```python
from build123d import *

# Parameters (mm, degrees)
SKETCH_1_W                = 180
SKETCH_1_H                = 43
EXTRUDE_335_DEPTH         = 4
SKETCH_2_R                = 5.1
SKETCH_2_R_2              = 1.6
CUT_EXTRUDE_616_DEPTH     = 5
SKETCH_10_W               = 20
SKETCH_10_H               = 43
CUT_EXTRUDE_3591_DEPTH    = 5
SKETCH_11_W               = 18
SKETCH_11_H               = 43
EXTRUDE_3904_DEPTH        = 4
SKETCH_12_W               = 40
SKETCH_12_H               = 13
CUT_EXTRUDE_3_DEPTH       = 10
SKETCH_14_R               = 1.6
CUT_EXTRUDE_4861_DEPTH    = 10
SKETCH_15_R               = 1.6
CUT_EXTRUDE_5298_DEPTH    = 5
PATTERN_LINEAR_5588_COUNT = 2
PATTERN_LINEAR_5588_PITCH = 29.8
CUT_EXTRUDE_6381_DEPTH    = 5
SKETCH_19_W               = 104
SKETCH_19_H               = 43
CUT_EXTRUDE_7034_DEPTH    = 5
FILLET_9_R                = 5
CUT_EXTRUDE_1_DEPTH       = 5
SKETCH_30_W               = 2
SKETCH_30_H               = 43
EXTRUDE_1_DEPTH           = 4
SKETCH_32_W               = 9
SKETCH_32_H               = 43
EXTRUDE_2_DEPTH           = 4
FILLET_11_R               = 5
EXTRUDE_3_DEPTH           = 4
FILLET_12_R               = 5
SKETCH_34_R               = 1.500000001
SKETCH_34_R_2             = 1.500000004
CUT_EXTRUDE_3_2_DEPTH     = 5
SKETCH_35_R               = 1.6
CUT_EXTRUDE_4_DEPTH       = 5
SKETCH_36_R               = 1.6
CUT_EXTRUDE_5_DEPTH       = 5
SKETCH_37_R               = 1.6
CUT_EXTRUDE_6_DEPTH       = 5
CUT_EXTRUDE_7_DEPTH       = 5
FILLET_15_R               = 1


with BuildPart() as part:
    # 草图1 → Extrude 335 (new body)
    with BuildSketch(Plane(origin=(0, 0, 0), x_dir=(1, 0, 0), z_dir=(0, 1, 0))):
        Rectangle(SKETCH_1_W, SKETCH_1_H)
    extrude(amount=EXTRUDE_335_DEPTH)

    # 草图2 → Cut-Extrude 616 (cut, through all)
    with BuildSketch(Plane(origin=(0, 4, 0), x_dir=(1, 0, 0), z_dir=(0, 1, 0))):
        with Locations((55, -5)):
            Circle(SKETCH_2_R)
        with Locations((63, -5)):
            Circle(SKETCH_2_R_2)
        with Locations((55, -13)):
            Circle(SKETCH_2_R_2)
        with Locations((47, -5)):
            Circle(SKETCH_2_R_2)
        with Locations((55, 3)):
            Circle(SKETCH_2_R_2)
    extrude(amount=-CUT_EXTRUDE_616_DEPTH, mode=Mode.SUBTRACT)

    # 草图10 → Cut-Extrude 3591 (cut, through all)
    with BuildSketch(Plane(origin=(0, 4, 0), x_dir=(1, 0, 0), z_dir=(0, 1, 0))):
        with Locations((80, 0)):
            Rectangle(SKETCH_10_W, SKETCH_10_H)
    extrude(amount=-CUT_EXTRUDE_3591_DEPTH, mode=Mode.SUBTRACT)

    # 草图11 → Extrude 3904 (add, through all)
    with BuildSketch(Plane(origin=(0, 4, 0), x_dir=(1, 0, 0), z_dir=(0, 1, 0))):
        with Locations((-99, 0)):
            Rectangle(SKETCH_11_W, SKETCH_11_H)
    extrude(amount=-EXTRUDE_3904_DEPTH)

    # 草图12 → Cut-Extrude 3 (cut)
    with BuildSketch(Plane(origin=(0, 4, 0), x_dir=(1, 0, 0), z_dir=(0, 1, 0))):
        with Locations((-88, -21.5)):
            Rectangle(SKETCH_12_W, SKETCH_12_H)
    extrude(amount=-CUT_EXTRUDE_3_DEPTH, mode=Mode.SUBTRACT)

    # 草图14 → Cut-Extrude 4861 (cut)
    with BuildSketch(Plane(origin=(0, 4, 0), x_dir=(1, 0, 0), z_dir=(0, 1, 0))):
        with Locations((46, -18.5)):
            Circle(SKETCH_14_R)
        with Locations((64, -18.5)):
            Circle(SKETCH_14_R)
    extrude(amount=-CUT_EXTRUDE_4861_DEPTH, mode=Mode.SUBTRACT)

    # 草图15 → Cut-Extrude 5298 (cut, through all)
    with BuildSketch(Plane(origin=(0, 4, 0), x_dir=(1, 0, 0), z_dir=(0, 1, 0))):
        with Locations((-102.9, 3.25)):
            Circle(SKETCH_15_R)
        with Locations((-73.1, 3.25)):
            Circle(SKETCH_15_R)
    extrude(amount=-CUT_EXTRUDE_5298_DEPTH, mode=Mode.SUBTRACT)

    # 草图16 → Cut-Revolve 5530 (revolve, cut)
    with BuildSketch(Plane.XY.offset(-3.25)):
        Polygon((-102.9, 0), (-99.7, 0), (-101.3, 1.6), (-102.9, 1.6), align=None)
    cut_revolve_5530 = revolve(axis=Axis((-102.9, -994.071718491, -3.25), (0, 1, 0)), mode=Mode.SUBTRACT)

    # Pattern Linear 5588: Cut-Revolve 5530 ×2
    with Locations(*[(i * PATTERN_LINEAR_5588_PITCH, 0, 0) for i in range(1, PATTERN_LINEAR_5588_COUNT)]):
        add(cut_revolve_5530, mode=Mode.SUBTRACT)

    # 草图17 → Cut-Extrude 6381 (cut, through all)
    with BuildSketch(Plane.XZ):
        with BuildLine():
            Line((-104.45, 3.75), (-101.35, 3.75))
            ThreePointArc((-101.35, 3.75), (-99.85, 5.25), (-101.35, 6.75))
            Line((-101.35, 6.75), (-101.35, 9.75))
            ThreePointArc((-101.35, 9.75), (-99.85, 11.25), (-101.35, 12.75))
            Line((-101.35, 12.75), (-104.45, 12.75))
            ThreePointArc((-104.45, 12.75), (-105.95, 11.25), (-104.45, 9.75))
            Line((-104.45, 9.75), (-104.45, 6.75))
            ThreePointArc((-104.45, 6.75), (-105.95, 5.25), (-104.45, 3.75))
        make_face()
        with BuildLine():
            Line((-104.45, -16.25), (-104.45, -13.25))
            ThreePointArc((-104.45, -13.25), (-105.95, -11.75), (-104.45, -10.25))
            Line((-104.45, -10.25), (-101.35, -10.25))
            ThreePointArc((-101.35, -10.25), (-99.85, -11.75), (-101.35, -13.25))
            Line((-101.35, -13.25), (-101.35, -16.25))
            ThreePointArc((-101.35, -16.25), (-99.85, -17.75), (-101.35, -19.25))
            Line((-101.35, -19.25), (-104.45, -19.25))
            ThreePointArc((-104.45, -19.25), (-105.95, -17.75), (-104.45, -16.25))
        make_face()
        with BuildLine():
            Line((-71.55, -16.25), (-71.55, -13.25))
            ThreePointArc((-71.55, -13.25), (-70.05, -11.75), (-71.55, -10.25))
            Line((-71.55, -10.25), (-74.65, -10.25))
            ThreePointArc((-74.65, -10.25), (-76.15, -11.75), (-74.65, -13.25))
            Line((-74.65, -13.25), (-74.65, -16.25))
            ThreePointArc((-74.65, -16.25), (-76.15, -17.75), (-74.65, -19.25))
            Line((-74.65, -19.25), (-71.55, -19.25))
            ThreePointArc((-71.55, -19.25), (-70.05, -17.75), (-71.55, -16.25))
        make_face()
        with BuildLine():
            Line((-71.55, 9.75), (-71.55, 6.75))
            ThreePointArc((-71.55, 6.75), (-70.05, 5.25), (-71.55, 3.75))
            Line((-71.55, 3.75), (-74.65, 3.75))
            ThreePointArc((-74.65, 3.75), (-76.15, 5.25), (-74.65, 6.75))
            Line((-74.65, 6.75), (-74.65, 9.75))
            ThreePointArc((-74.65, 9.75), (-76.15, 11.25), (-74.65, 12.75))
            Line((-74.65, 12.75), (-71.55, 12.75))
            ThreePointArc((-71.55, 12.75), (-70.05, 11.25), (-71.55, 9.75))
        make_face()
    extrude(amount=-CUT_EXTRUDE_6381_DEPTH, mode=Mode.SUBTRACT)

    # 草图19 → Cut-Extrude 7034 (cut, through all)
    with BuildSketch(Plane(origin=(0, 4, 0), x_dir=(1, 0, 0), z_dir=(0, 1, 0))):
        with Locations((-56, 0)):
            Rectangle(SKETCH_19_W, SKETCH_19_H)
    extrude(amount=-CUT_EXTRUDE_7034_DEPTH, mode=Mode.SUBTRACT)

    # 圆角9
    fillet_9_edges = [part.edges().sort_by_distance(p)[0] for p in [
        (-4, 2, 21.5),
        (-4, 2, -21.5),
        (70, 2, 21.5),
        (70, 2, -21.5),
    ]]
    fillet(fillet_9_edges, radius=FILLET_9_R)

    # 草图29 → Cut-Extrude 1 (cut, through all)
    with BuildSketch(Plane(origin=(0, 4, 0), x_dir=(1, 0, 0), z_dir=(0, 1, 0))):
        Polygon((1, 21.5), (10.830690118, 21.5), (10.830690118, -21.5), (1, -21.5), (-4.254253264, -21.5), (-4.254253264, 21.5), align=None)
    extrude(amount=-CUT_EXTRUDE_1_DEPTH, mode=Mode.SUBTRACT)

    # 草图30 → 凸台-拉伸1 (add)
    with BuildSketch(Plane(origin=(0, 4, 0), x_dir=(1, 0, 0), z_dir=(0, 1, 0))):
        with Locations((9.830690118, 0)):
            Rectangle(SKETCH_30_W, SKETCH_30_H)
    extrude(amount=-EXTRUDE_1_DEPTH)

    # 草图32 → Extrude 2 (add)
    with BuildSketch(Plane.XZ):
        with Locations((4.330690118, 0)):
            Rectangle(SKETCH_32_W, SKETCH_32_H)
    extrude(amount=-EXTRUDE_2_DEPTH)

    # 圆角11
    fillet_11_edges = [part.edges().sort_by_distance(p)[0] for p in [
        (-0.169309882, 2, -21.5),
        (-0.169309882, 2, 21.5),
    ]]
    fillet(fillet_11_edges, radius=FILLET_11_R)

    # 草图33 → 凸台-拉伸3 (add)
    with BuildSketch(Plane.XZ):
        Polygon((70, 16.5), (70, 25.500000005), (65, 25.500000005), (0, 25.500000005), (-0.169309882, 25.500000005), (-0.169309882, 16.5), align=None)
    extrude(amount=-EXTRUDE_3_DEPTH)

    # 圆角12
    fillet_12_edges = [part.edges().sort_by_distance(p)[0] for p in [
        (-0.169309882, 2, 25.500000005),
        (70, 2, 25.500000005),
    ]]
    fillet(fillet_12_edges, radius=FILLET_12_R)

    # 草图34 → Cut-Extrude 3 2 (cut, through all)
    with BuildSketch(Plane.XZ):
        with Locations((63.455393867, 20.5)):
            Circle(SKETCH_34_R)
        with Locations((47.301465353, 20.5)):
            Circle(SKETCH_34_R_2)
    extrude(amount=-CUT_EXTRUDE_3_2_DEPTH, mode=Mode.SUBTRACT)

    # 草图35 → 切除-拉伸4 (cut, through all)
    with BuildSketch(Plane.XZ):
        with Locations((34, 0.636740591)):
            Circle(SKETCH_35_R)
        with Locations((34, 9.1)):
            Circle(SKETCH_35_R)
    extrude(amount=-CUT_EXTRUDE_4_DEPTH, mode=Mode.SUBTRACT)

    # 草图36 → 切除-拉伸5 (cut, through all)
    with BuildSketch(Plane.XZ):
        with Locations((9.830690118, -5.9)):
            Circle(SKETCH_36_R)
        with Locations((9.830690118, 9.7)):
            Circle(SKETCH_36_R)
        with Locations((9.830690118, -16.948915218)):
            Circle(SKETCH_36_R)
        with Locations((19.830690118, -16.948915218)):
            Circle(SKETCH_36_R)
    extrude(amount=-CUT_EXTRUDE_5_DEPTH, mode=Mode.SUBTRACT)

    # 草图37 → 切除-拉伸6 (cut, through all)
    with BuildSketch(Plane(origin=(0, 4, 0), x_dir=(1, 0, 0), z_dir=(0, 1, 0))):
        with Locations((19.925091374, -9.664193429)):
            Circle(SKETCH_37_R)
    extrude(amount=-CUT_EXTRUDE_6_DEPTH, mode=Mode.SUBTRACT)

    # 草图38 → 切除-拉伸7 (cut, through all)
    with BuildSketch(Plane.XZ):
        with BuildLine():
            Line((44, 25.500000005), (44, 19.500000005))
            ThreePointArc((44, 19.500000005), (43.414213562, 18.085786442), (42, 17.500000005))
            Line((42, 17.500000005), (26, 17.500000005))
            ThreePointArc((26, 17.500000005), (24.585786438, 18.085786442), (24, 19.500000005))
            Line((24, 19.500000005), (24, 25.500000005))
            Line((24, 25.500000005), (44, 25.500000005))
        make_face()
    extrude(amount=-CUT_EXTRUDE_7_DEPTH, mode=Mode.SUBTRACT)

    # 圆角15
    fillet_15_edges = [part.edges().sort_by_distance(p)[0] for p in [
        (24, 2, 25.500000005),
        (44, 2, 25.500000005),
    ]]
    fillet(fillet_15_edges, radius=FILLET_15_R)


solid = part.part
```
Design review of the part built by this model. Coordinates are the model's own, in mm. A direction names the side the tool comes from. Round coordinates to 2 decimals unless told otherwise and drop trailing zeros. Write each loop counter-clockwise with the first axis right and the second up, starting at its lowest first coordinate (ties: lowest second). Pieces come first, ordered by that corner, then holes. Notation, with made-up numbers: (31, 5.25) -> (52, 5.25) arc R24 cw to (52, 24.25) -> close; hole circle Ø3 at (33, -27). An arc over 180 degrees is marked (long way). Answer in a Markdown table with one row per item.
Q1. Take a section at A-A, the plane x = 34. State the section outline as (y, z) points.
The answers:
| item | result |
|---|---|
| outline | (0, -21.5) -> (4, -21.5) -> (4, -0.96) -> (0, -0.96) -> close; (0, 2.24) -> (4, 2.24) -> (4, 7.5) -> (0, 7.5) -> close; (0, 10.7) -> (4, 10.7) -> (4, 17.5) -> (0, 17.5) -> close |
Q2. Take a section at D-D, the plane z = 13. State the section outline as (x, y) points, then the cut area to 3 significant figures.
The answers:
| item | result |
|---|---|
| outline | (-0.17, 0) -> (53.4, 0) -> (53.4, 4) -> (-0.17, 4) -> close; (56.6, 0) -> (70, 0) -> (70, 4) -> (56.6, 4) -> close |
| area | 268 mm² |
Q3. For faces 1 (the face through (68.57, 2.03, 24)), 2 (the face through (24.6, 1.97, 18.07)), list the 3-axis set-ups (+Z, -Z, +X, -X, +Y, -Y) from which the entire face can be reached by the end or side of a thin tool; tool diameter is ignored.
The answers:
| item | result |
|---|---|
| face 1 | +Z, +X, +Y, -Y |
| face 2 | +Z, +Y, -Y |
Q4. Draft analysis for pull direction Z (two halves, no side actions). For faces 3 (the face through (14, 2, 25.5)), 4 (the face through (44, 2, 22)), 5 (the face through (56.48, 2.03, -2.39)), 6 (the face through (32.4, 2, 0.7)), state which applies: +Z half, -Z half, draft (parallel to the pull), parting line (faces both ways), or undercut.
The answers:
| item | result |
|---|---|
| face 3 | +Z half |
| face 4 | draft |
| face 5 | undercut |
| face 6 | undercut |
Q5. Take a section at B-B, the plane z = 5. State the section outline as (x, y) points.
The answers:
| item | result |
|---|---|
| outline | (-0.17, 0) -> (45.4, 0) -> (45.4, 4) -> (-0.17, 4) -> close; (48.6, 0) -> (49.9, 0) -> (49.9, 4) -> (48.6, 4) -> close; (60.1, 0) -> (61.4, 0) -> (61.4, 4) -> (60.1, 4) -> close; (64.6, 0) -> (70, 0) -> (70, 4) -> (64.6, 4) -> close |
Q6. Clearance check with a flat-ended pin moving along its axis: pin 1 Ø1.2 at (x, y) = (37, 1.5) entering from +Z. State where the tip first meets the part, or that it passes through.
The answers:
| item | result |
|---|---|
| pin 1 | z = 17.5 |
Q7. To check wall thickness, follow L1, parallel to X at y = 2.1, z = 5; L2, parallel to X at y = 1.6, z = 13; L3, parallel to X at y = 0.95, z = 21. State the ranges of each line that lie inside material, in increasing order. Write a range as [from, to].
The answers:
| item | result |
|---|---|
| L1 | [-0.17, 45.4], [48.6, 49.9], [60.1, 61.4], [64.6, 70] |
| L2 | [-0.17, 53.4], [56.6, 70] |
| L3 | [-0.14, 24], [44, 45.89], [48.72, 62.04], [64.87, 69.97] |
Q8. Take a section at C-C, the plane x = 55. State the section outline as (y, z) points, then the cut area to 3 significant figures.
The answers:
| item | result |
|---|---|
| outline | (0, -21.5) -> (4, -21.5) -> (4, -4.6) -> (0, -4.6) -> close; (0, -1.4) -> (4, -1.4) -> (4, -0.1) -> (0, -0.1) -> close; (0, 10.1) -> (4, 10.1) -> (4, 11.4) -> (0, 11.4) -> close; (0, 14.6) -> (4, 14.6) -> (4, 25.5) -> (0, 25.5) -> close |
| area | 122 mm² |
